Input: part model. Units: mm. Frame: model coordinates. Face numbers are marked on the shaded views. A direction names the side the tool comes from. Round coordinates to 2 decimals unless told otherwise and drop trailing zeros. Loops run counter-clockwise (first coordinate to the right, second up) from the corner with the lowest first, then second, coordinate; pieces in that order, holes last. Notation, with made-up numbers: M 9,-26 L 54,-26 A4 cw 54,-20 Z; hole C -28.5,31 d4. An arc over 180 degrees is marked long. Put each result on its own line as item: value. Start each with the question number.
1) Pin query (flat end, axial travel): pin 1 (3 mm diameter, centred on x = -2.5, y = 4, fed in from -Z); pin 2 (4 mm diameter, centred on x = -7, z = -24, fed in from +Y); pin 3 (2 mm diameter, centred on x = 0.5, z = 0, fed in from +Y). Return the tip coordinate at first contact, or that it passes through.
2) Line query: probe 1 along Y at (x, z) = (-6.35, 0); probe 2 along Y at (x, z) = (6.3, 0); probe 3 along Y at (x, z) = (8.4, 0). Output: solid intervals per line, ascending.
3) Section B-B on y = 6. Output: boundary loops of the cut face in (x, z) (3 decimals), plus the area to 3 significant figures.
4) Draft query along Y for the marked faces 4, 5 and 6. Return one class per face: +Y half, -Y half, draft (parallel to the pull), parting line (faces both ways), or undercut.
5) Section A-A on z = 31. Output: boundary loops of the cut face in (x, y), plus the area to 3 significant figures.
6) Reachability of the marked faces 1, 2 and 3 from +Z, -Z, +X, -X, +Y, -Y: full face, straight path, thin tool, end or side. Return the list, or none.
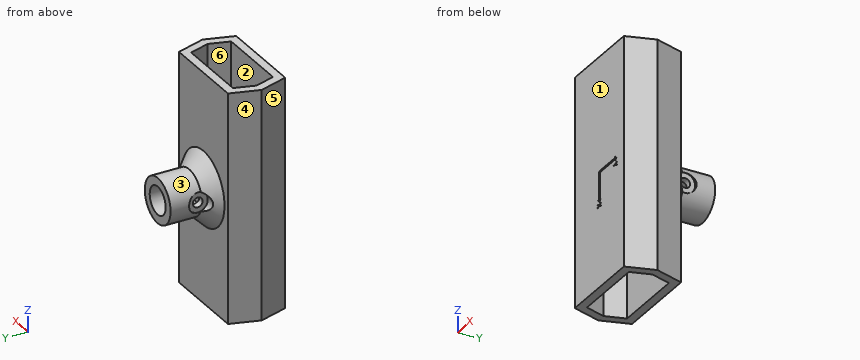
from build123d import *

# Parameters (mm, degrees)
EXTRUDE_1_DEPTH          = 40
CUT_EXTRUDE_3_DEPTH      = 81
CHAMFER_1_SIZE           = 5
SKETCH_5_R               = 1.7
CUT_EXTRUDE_1_DEPTH      = 10
CUT_EXTRUDE_1_DEPTH_BACK = 10
SKETCH_6_R               = 3.5
CUT_EXTRUDE_2_DEPTH      = 10
CUT_EXTRUDE_4_DEPTH      = 0.6
CUT_EXTRUDE_5_DEPTH      = 0.6
SKETCH_10_R              = 0.90757886
CUT_EXTRUDE_6_DEPTH      = 1


with BuildPart() as part:
    # Sketch 1 → Extrude 1 (new body, symmetric)
    with BuildSketch(Plane.XY):
        Polygon((-15, 0), (15, 0), (18.130448736, -10), (15, -20), (-15, -20), (-18.130448736, -10), align=None)
    extrude(amount=EXTRUDE_1_DEPTH, both=True)

    # Sketch 7 → Cut-Extrude 3 (cut, through all)
    with BuildSketch(Plane(origin=(0, 0, -40), x_dir=(-1, 0, 0), z_dir=(0, 0, -1))):
        Polygon((14.986888042, -10), (12.795573927, -3), (-12.795573927, -3), (-14.986888042, -10), (-12.795573927, -17), (12.795573927, -17), align=None)
    extrude(amount=-CUT_EXTRUDE_3_DEPTH, mode=Mode.SUBTRACT)

    # Sketch 3 → Revolve 1 (revolve)
    with BuildSketch(Plane.XY):
        Polygon((4.875, 16), (7.875, 16), (7.875, 0), (0, 0), (0, 2), (4.875, 2), align=None)
    revolve(axis=Axis((0, 0, 0), (0, 1, 0)))

    # Chamfer 1
    chamfer_1_edges = [part.edges().sort_by_distance(p)[0] for p in [
        (-7.875, 0, 0),
    ]]
    chamfer(chamfer_1_edges, length=CHAMFER_1_SIZE)

    # Sketch 5 → Cut-Extrude 1 (cut, two sides)
    with BuildSketch(Plane(origin=(0, 0, 0), x_dir=(0, 0, -1), z_dir=(1, 0, 0))) as cut_extrude_1_sk:
        with Locations((0, 6)):
            Circle(SKETCH_5_R)
    extrude(amount=CUT_EXTRUDE_1_DEPTH, mode=Mode.SUBTRACT)
    extrude(cut_extrude_1_sk.sketch, amount=-CUT_EXTRUDE_1_DEPTH_BACK, mode=Mode.SUBTRACT)

    # Sketch 6 → Cut-Extrude 2 (cut)
    with BuildSketch(Plane(origin=(7, 0, 0), x_dir=(0, 0, -1), z_dir=(1, 0, 0))):
        with Locations((0, 6)):
            Circle(SKETCH_6_R)
    cut_extrude_2 = extrude(amount=CUT_EXTRUDE_2_DEPTH, mode=Mode.SUBTRACT)

    # Mirror 1: Cut-Extrude 2 across plane
    add(cut_extrude_2.mirror(Plane(origin=(0, 0, 0), x_dir=(0, 0, 1), z_dir=(1, 0, 0))), mode=Mode.SUBTRACT)

    # Sketch 8 → Cut-Extrude 4 (cut)
    with BuildSketch(Plane.XZ.offset(20)):
        Polygon((-0.3, 0), (-0.3, -9.488320233), (-0.9, -9.488320233), (0, -10.399776511), (0.9, -9.488320233), (0.3, -9.488320233), (0.3, 0), align=None)
        Polygon((0, -0.3), (9.488320233, -0.3), (9.488320233, -0.9), (10.399776511, 0), (9.488320233, 0.9), (9.488320233, 0.3), (0, 0.3), align=None)
    extrude(amount=-CUT_EXTRUDE_4_DEPTH, mode=Mode.SUBTRACT)

    # Sketch 9 → Cut-Extrude 5 (cut)
    with BuildSketch(Plane.XZ.offset(20)):
        Polygon((1.036018744, -10.883097159), (1.036018744, -11.163798913), (0.217305293, -11.561459732), (1.036018744, -11.959120551), (1.036018744, -12.239822305), (-0.016612835, -11.690114703), (-0.963981256, -12.181342773), (-0.963981256, -11.900641018), (-0.238835058, -11.561459732), (-0.963981256, -11.222278445), (-0.963981256, -10.941576691), (-0.016612835, -11.432804761), align=None)
        Polygon((10.812249856, -2.737510211), (9.712834652, -2.187802609), (8.812249856, -2.187802609), (8.812249856, -1.918796761), (9.712834652, -1.918796761), (10.812249856, -1.369089158), (10.812249856, -1.638095006), (9.958448687, -2.047451731), (9.958448687, -2.059147638), (10.812249856, -2.468504363), align=None)
    extrude(amount=-CUT_EXTRUDE_5_DEPTH, mode=Mode.SUBTRACT)

    # Sketch 10 → Cut-Extrude 6 (cut)
    with BuildSketch(Plane(origin=(0, 2, 0), x_dir=(1, 0, 0), z_dir=(0, 1, 0))):
        Circle(SKETCH_10_R)
    extrude(amount=-CUT_EXTRUDE_6_DEPTH, mode=Mode.SUBTRACT)


solid = part.part
Geometry results:
1. pin 1: stops at z = -10.11
1. pin 2: stops at y = 0
1. pin 3: stops at y = 2
2. probe 1: y = -20 to -17, -3 to 4.3, 7.7 to 16
2. probe 2: y = -19.4 to -17, -3 to 4.3, 7.7 to 16
2. probe 3: y = -19.4 to -17, -3 to 2.5
3. outline: M -7.054,-3.5 A7.875 ccw 7.054,-3.5 L 7,-3.5 L 7,-1.7 L 4.569,-1.7 A4.875 cw -4.569,-1.7 L -7,-1.7 L -7,-3.5 Z; M -7.054,3.5 L -7,3.5 L -7,1.7 L -4.569,1.7 A4.875 cw 4.569,1.7 L 7,1.7 L 7,3.5 L 7.054,3.5 A7.875 ccw Z
3. area: 96.5 mm²
4. face 4: +Y half
4. face 5: -Y half
4. face 6: undercut
5. outline: M -18.13,-10 L -15,-20 L 15,-20 L 18.13,-10 L 15,0 L -15,0 Z; hole M -14.99,-10 L -12.8,-17 L 12.8,-17 L 14.99,-10 L 12.8,-3 L -12.8,-3 Z
5. area: 274 mm²
6. face 1: +Z, -Z, +X, -X, -Y
6. face 2: +Z, -Z
6. face 3: +Y
